Read the model definition and answer for the solid it produces. Units are mm, in the model's axes. A direction names the side the tool comes from. Round coordinates to 2 decimals unless told otherwise and drop trailing zeros. Order: outer loops, then holes, each group sorted by start corner. A loop starts at its lowest first (then second) coordinate and runs counter-clockwise, first axis right, second up. Notation, with made-up numbers: M -4.75,-6.75 L 35.25,-6.75 A28 ccw 35.25,13.25 Z; hole C 60,68 d9. An arc over 180 degrees is marked long. Use one line per item in the form item = value. Start each with the question number.
from build123d import *

# Parameters (mm, degrees)
SKETCH_1_W          = 62
SKETCH_1_H          = 46
EXTRUDE_1_DEPTH     = 15
SKETCH_2_W          = 58
SKETCH_2_H          = 42
CUT_EXTRUDE_1_DEPTH = 10
CUT_EXTRUDE_2_REACH = 69.809
SKETCH_3_W          = 12
SKETCH_3_H          = 20
CUT_EXTRUDE_3_REACH = 57.875
SKETCH_5_W          = 36
SKETCH_5_H          = 10
CUT_EXTRUDE_4_REACH = 57.875
SKETCH_6_W          = 20
SKETCH_6_H          = 10
SKETCH_7_R          = 1.5
CUT_EXTRUDE_5_DEPTH = 40.874804075
SKETCH_8_R          = 2
CUT_EXTRUDE_6_DEPTH = 3


with BuildPart() as part:
    # 草图1 → 凸台-拉伸1 (new body)
    with BuildSketch(Plane(origin=(0, 0, 0), x_dir=(1, 0, 0), z_dir=(0, 1, 0))):
        Rectangle(SKETCH_1_W, SKETCH_1_H)
    extrude(amount=EXTRUDE_1_DEPTH)

    # 草图2 → 切除-拉伸1 (cut)
    with BuildSketch(Plane(origin=(0, 15, 0), x_dir=(1, 0, 0), z_dir=(0, 1, 0))):
        Rectangle(SKETCH_2_W, SKETCH_2_H)
    extrude(amount=-CUT_EXTRUDE_1_DEPTH, mode=Mode.SUBTRACT)

    # 草图3 → 切除-拉伸2 (cut, up to next)
    with BuildSketch(Plane.ZY.offset(31), mode=Mode.PRIVATE) as cut_extrude_2_sk1:
        with Locations((0, 15)):
            Rectangle(SKETCH_3_W, SKETCH_3_H)
    cut_extrude_2_tool1 = extrude(cut_extrude_2_sk1.sketch, amount=-CUT_EXTRUDE_2_REACH, mode=Mode.PRIVATE) & part.part
    add(cut_extrude_2_tool1.solids().sort_by_distance((-31, 15, 0))[0], mode=Mode.SUBTRACT)

    # 草图5 → 切除-拉伸3 (cut, up to next)
    with BuildSketch(Plane.XY.offset(-21), mode=Mode.PRIVATE) as cut_extrude_3_sk1:
        with Locations((11, 10)):
            Rectangle(SKETCH_5_W, SKETCH_5_H)
    cut_extrude_3_tool1 = extrude(cut_extrude_3_sk1.sketch, amount=-CUT_EXTRUDE_3_REACH, mode=Mode.PRIVATE) & part.part
    add(cut_extrude_3_tool1.solids().sort_by_distance((11, 10, -21))[0], mode=Mode.SUBTRACT)

    # 草图6 → 切除-拉伸4 (cut, up to next)
    with BuildSketch(Plane(origin=(0, 0, 21), x_dir=(-1, 0, 0), z_dir=(0, 0, -1)), mode=Mode.PRIVATE) as cut_extrude_4_sk1:
        with Locations((-19, 10)):
            Rectangle(SKETCH_6_W, SKETCH_6_H)
    cut_extrude_4_tool1 = extrude(cut_extrude_4_sk1.sketch, amount=-CUT_EXTRUDE_4_REACH, mode=Mode.PRIVATE) & part.part
    add(cut_extrude_4_tool1.solids().sort_by_distance((19, 10, 21))[0], mode=Mode.SUBTRACT)

    # 草图7 → 切除-拉伸5 (cut, through all)
    with BuildSketch(Plane(origin=(0, 5, 0), x_dir=(1, 0, 0), z_dir=(0, 1, 0))):
        with Locations(Location((26, -18, 0), (0, 0, 270))):
            Circle(SKETCH_7_R)
        with Locations(Location((26, 18, 0), (0, 0, 270))):
            Circle(SKETCH_7_R)
        with Locations(Location((-10, 18, 0), (0, 0, 270))):
            Circle(SKETCH_7_R)
        with Locations(Location((-10, -18, 0), (0, 0, 270))):
            Circle(SKETCH_7_R)
    extrude(amount=-CUT_EXTRUDE_5_DEPTH, mode=Mode.SUBTRACT)

    # 草图8 → 切除-拉伸6 (cut)
    with BuildSketch(Plane.XZ):
        with Locations(Location((-10, 18, 0), (0, 0, 270))):
            Circle(SKETCH_8_R)
        with Locations(Location((26, 18, 0), (0, 0, 270))):
            Circle(SKETCH_8_R)
        with Locations(Location((26, -18, 0), (0, 0, 270))):
            Circle(SKETCH_8_R)
        with Locations(Location((-10, -18, 0), (0, 0, 270))):
            Circle(SKETCH_8_R)
    extrude(amount=-CUT_EXTRUDE_6_DEPTH, mode=Mode.SUBTRACT)


solid = part.part
Item 1: Section B-B (y = 13.5) is taken. Write down the section's boundary in (x, z).
Item 2: Section A-A (z = 18) is taken. Write down the section's boundary in (x, y).
Item 3: Find the intervals of material crossed by L1, parallel to X at y = 1.1, z = 18; L2, parallel to X at y = 9.75, z = -11; L3, parallel to Z at x = -11, y = 5.25, in increasing order. Write a range as [from, to].
Item 4: Section D-D (z = 10.5) is taken. Write down the section's boundary in (x, y), and give its area (3 significant figures).
Item 5: Given P1, Ø2, axis at x = -10.5, z = 17.5, coming from the -Y side; P2, Ø5, axis at x = -10, z = -18, coming from the +Y side, each flat-ended and moving along its own axis, determine where each tip first touches the part or whether it passes through.
Item 6: A tool of negligible diameter and unlimited length cuts with its end or side. For faces 4 (the flat face through (9, 10, 22)), 5 (the flat face through (-29, 10, -13)), 6 (the cylindrical face through (24, 1, 18)), from which of +Z, -Z, +X, -X, +Y, -Y can it reach the whole face along a straight path? Write none if from no direction.
Item 7: For a pull along X with two mould halves and no side action, classify faces 1 (the flat face through (-7, 10, -22)), 2 (the flat face through (-24.4, 15, -21.5)), 3 (the flat face through (-31, 4, 0)) as pulls with the +X half, pulls with the -X half, needs draft (parallel to the pull), parting line crosses it, or undercut.
Item 8: Section C-C (x = -15) is taken. Write down the section's boundary in (y, z).
The answers:
q1.outline = M -31,-23 L -7,-23 L -7,-21 L -29,-21 L -29,-6 L -31,-6 Z; M -31,6 L -29,6 L -29,21 L 9,21 L 9,23 L -31,23 Z; M 29,-23 L 31,-23 L 31,23 L 29,23 Z
q2.outline = M -31,0 L -12,0 L -12,3 L -11.5,3 L -11.5,5 L -29,5 L -29,15 L -31,15 Z; M -8.5,3 L -8,3 L -8,0 L 24,0 L 24,3 L 24.5,3 L 24.5,5 L -8.5,5 Z; M 27.5,3 L 28,3 L 28,0 L 31,0 L 31,15 L 29,15 L 29,5 L 27.5,5 Z
q3.L1 = [-31, -12], [-8, 24], [28, 31]
q3.L2 = [-31, -29], [29, 31]
q3.L3 = [-23, -21], [21, 23]
q4.outline = M -31,0 L 31,0 L 31,15 L 29,15 L 29,5 L -29,5 L -29,15 L -31,15 Z
q4.area = 350 mm²
q5.P1 = 3
q5.P2 = 5
q6.face_4 = +Z, -Z, +Y
q6.face_5 = +Y
q6.face_6 = -Y
q7.face_1 = undercut
q7.face_2 = needs draft
q7.face_3 = pulls with the -X half
q8.outline = M 0,-23 L 15,-23 L 15,-21 L 5,-21 L 5,21 L 15,21 L 15,23 L 0,23 Z
